The model under review builds one solid part; all positions refer to its coordinate system, in mm. Face numbers are marked on the shaded views. A direction names the side the tool comes from. Round coordinates to 2 decimals unless told otherwise and drop trailing zeros. Order: outer loops, then holes, each group sorted by start corner. A loop starts at its lowest first (then second) coordinate and runs counter-clockwise, first axis right, second up. Notation, with made-up numbers: M 14.5,66.25 L 21.5,66.25 A20 cw 21.5,100.25 Z; hole C 14,-13 d5. An arc over 180 degrees is marked long. One line per item, written item: value. Start each with the question number.
from build123d import *

# Parameters (mm, degrees)
SKETCH1_W           = 28
SKETCH1_H           = 28
BOSS_EXTRUDE1_DEPTH = 6
SKETCH2_R           = 6
BOSS_EXTRUDE2_DEPTH = 6
SKETCH3_R           = 2.4
CUT_EXTRUDE1_DEPTH  = 49.456165758
CUT_EXTRUDE2_DEPTH  = 10
SKETCH5_R           = 1.4
CUT_EXTRUDE3_DEPTH  = 10
CUT_EXTRUDE4_START  = 10
SKETCH6_R           = 1.4
CUT_EXTRUDE4_DEPTH  = 10


with BuildPart() as part:
    # Sketch1 → Boss-Extrude1 (new body)
    with BuildSketch(Plane(origin=(0, 0, 0), x_dir=(1, 0, 0), z_dir=(0, 1, 0))):
        with Locations((14, 14)):
            Rectangle(SKETCH1_W, SKETCH1_H)
    extrude(amount=BOSS_EXTRUDE1_DEPTH)

    # Sketch2 → Boss-Extrude2 (add)
    with BuildSketch(Plane(origin=(0, 6, 0), x_dir=(1, 0, 0), z_dir=(0, 1, 0))):
        with Locations((0, 28)):
            Circle(SKETCH2_R)
        with Locations((28, 28)):
            Circle(SKETCH2_R)
        with Locations((28, 0)):
            Circle(SKETCH2_R)
        Circle(SKETCH2_R)
    extrude(amount=-BOSS_EXTRUDE2_DEPTH)

    # Sketch3 → Cut-Extrude1 (cut, through all)
    with BuildSketch(Plane(origin=(0, 6, 0), x_dir=(1, 0, 0), z_dir=(0, 1, 0))):
        with Locations(Location((0, 28, 0), (0, 0, 270))):
            Circle(SKETCH3_R)
        with Locations(Location((28, 28, 0), (0, 0, 90))):
            Circle(SKETCH3_R)
        with Locations(Location((28, 0, 0), (0, 0, 270))):
            Circle(SKETCH3_R)
        with Locations(Location((0, 0, 0), (0, 0, 90))):
            Circle(SKETCH3_R)
    extrude(amount=-CUT_EXTRUDE1_DEPTH, mode=Mode.SUBTRACT)

    # Sketch4 → Cut-Extrude2 (cut)
    with BuildSketch(Plane(origin=(0, 6, 0), x_dir=(1, 0, 0), z_dir=(0, 1, 0))):
        Polygon((11.878679656, 14), (3, 22.878679656), (3, 5.121320344), align=None)
        Polygon((22.878679656, 25), (5.121320344, 25), (14, 16.121320344), align=None)
        Polygon((25, 5.121320344), (25, 22.878679656), (16.121320344, 14), align=None)
        Polygon((14, 11.878679656), (5.121320344, 3), (22.878679656, 3), align=None)
    extrude(amount=-CUT_EXTRUDE2_DEPTH, mode=Mode.SUBTRACT)

    # Sketch5 → Cut-Extrude3 (cut)
    with BuildSketch(Plane(origin=(28, 0, 0), x_dir=(0, 0, -1), z_dir=(1, 0, 0))):
        with Locations(Location((0, 3, 0), (0, 0, 180))):
            Circle(SKETCH5_R)
        with Locations(Location((28, 3, 0), (0, 0, 180))):
            Circle(SKETCH5_R)
    extrude(amount=CUT_EXTRUDE3_DEPTH, mode=Mode.SUBTRACT)

    # Sketch6 → Cut-Extrude4 (cut)
    with BuildSketch(Plane.ZY.offset(CUT_EXTRUDE4_START)):
        with Locations((-28, 3)):
            Circle(SKETCH6_R)
        with Locations((0, 3)):
            Circle(SKETCH6_R)
    extrude(amount=-CUT_EXTRUDE4_DEPTH, mode=Mode.SUBTRACT)


solid = part.part
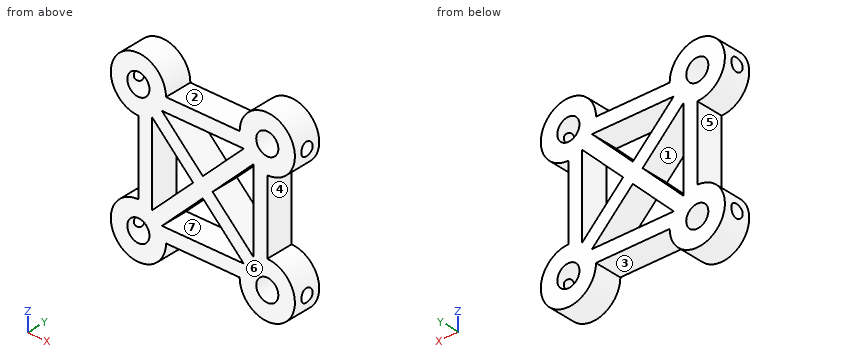
Item 1: Consider section A-A, the plane y = 0.75. Count the separate pieces of the cut face and the enclosed holes in it, then the cut area to 3 significant figures.
Item 2: Machinability: for the marked faces 1, 2 and 3, which of the approach directions +Z, -Z, +X, -X, +Y, -Y give a long, thin tool a straight path to every point of the face, cutting with its end or side? Answer none if there is none.
Item 3: Consider section C-C, the plane x = 29. Give the boundary of the cut face in (y, z), then the cut area to 3 significant figures.
Item 4: Consider section B-B, the plane z = -14.5. Give the boundary of the cut face in (x, y), then the cut area to 3 significant figures.
Item 5: Wall thickness on L1, parallel to X at y = 2.5, z = -20; L2, parallel to X at y = 2.5, z = 2; L3, parallel to Z at x = 19.5, y = 1.5: over which ranges is each line inside the solid? List them lowest first.
Item 6: Consider section D-D, the plane z = -9. Give the boundary of the cut face in (x, y), then the cut area to 3 significant figures.
Item 7: The part is to be moulded in two halves that separate along X. For the marked faces 4, 5, 6 and 7, say which applies: pulls with the +X half, pulls with the -X half, needs draft (parallel to the pull), parting line crosses it, or undercut.
Item 8: Clearance check with flat-ended pins moving along their axes: P1, Ø10, axis at x = 30, z = -27.5, coming from the -Y side; P2, Ø2, axis at y = 3, z = -28, coming from the -X side; P3, Ø2.5, axis at y = 3, z = 0, coming from the -X side; P4, Ø3, axis at y = 4, z = -14.5, coming from the -X side. State where each tip first meets the part, or that it passes through.
Computed:
1. separate pieces: 1
1. enclosed holes: 8
1. area: 736 mm^2
2. face 1: +Y, -Y
2. face 2: +Z, +Y, -Y
2. face 3: -Z, +Y, -Y
3. outline: M 0,-33.92 L 6,-33.92 L 6,-30.18 L 0,-30.18 Z; M 0,-25.82 L 6,-25.82 L 6,-22.08 L 0,-22.08 Z; M 0,-5.92 L 6,-5.92 L 6,-2.18 L 0,-2.18 Z; M 0,2.18 L 6,2.18 L 6,5.92 L 0,5.92 Z
3. area: 89.6 mm^2
4. outline: M 0,0 L 3,0 L 3,6 L 0,6 Z; M 11.38,0 L 16.62,0 L 16.62,6 L 11.38,6 Z; M 25,0 L 28,0 L 28,6 L 25,6 Z
4. area: 67.5 mm^2
5. L1: x = 0 to 3, 5.88 to 10.12, 17.88 to 22.12, 25 to 28
5. L2: x = -5.66 to -1.33, 1.33 to 5.66, 22.34 to 26.67, 29.33 to 33.66
5. L3: z = -28 to -25, -21.62 to -17.38, -10.62 to -6.38, -3 to 0
6. outline: M 0,0 L 3,0 L 3,6 L 0,6 Z; M 6.88,0 L 11.12,0 L 11.12,6 L 6.88,6 Z; M 16.88,0 L 21.12,0 L 21.12,6 L 16.88,6 Z; M 25,0 L 28,0 L 28,6 L 25,6 Z
6. area: 86.9 mm^2
7. face 4: pulls with the +X half
7. face 5: pulls with the -X half
7. face 6: needs draft
7. face 7: undercut
8. P1: stops at y = 0
8. P2: stops at x = 2.18
8. P3: stops at x = 2.05
8. P4: stops at x = 0
